Input: part model. Units: mm. Frame: model coordinates. A direction names the side the tool comes from. Round coordinates to 2 decimals unless told otherwise and drop trailing zeros. Loops run counter-clockwise (first coordinate to the right, second up) from the corner with the lowest first, then second, coordinate; pieces in that order, holes last. Notation, with made-up numbers: M 62.5,-23 L 120.5,-23 A13 ccw 120.5,-9 Z; hole C 37,40.5 d11. An arc over 180 degrees is marked long. Put each result on its own line as item: value. Start each with the question number.
1) Pin query (flat end, axial travel): pin 1 (5 mm diameter, centred on y = -0.5, z = -8, fed in from +X); pin 2 (2 mm diameter, centred on y = -3.5, z = -5.5, fed in from -X); pin 3 (5 mm diameter, centred on y = 4, z = -6, fed in from -X). Return the tip coordinate at first contact, or that it passes through.
2) Section C-C on x = -61.5. Output: boundary loops of the cut face in (y, z), plus the area to 3 significant figures.
3) Section A-A on y = 35. Output: boundary loops of the cut face in (x, z).
4) Reachability of faces 4 (the face through (-9.565, -40, -6)), 5 (the face through (-81, -3, -5)) from +Z, -Z, +X, -X, +Y, -Y: full face, straight path, thin tool, end or side. Return the list, or none.
5) Draft query along Y for faces 1 (the face through (-79, 20.744, -8)), 2 (the face through (-81, -38.396, -2)), 3 (the face through (-149.565, -40, -6)). Return one class per face: +Y half, -Y half, draft (parallel to the pull), parting line (faces both ways), or undercut.
6) Section D-D on z = -2.5. Output: boundary loops of the cut face in (x, y).
7) Section B-B on x = -84. Output: boundary loops of the cut face in (y, z).
8) Line query: probe 1 along Z at (x, y) = (-82, 14); probe 2 along Y at (x, z) = (-95.5, -3.5); probe 3 along Y at (x, z) = (-33, -7.5). Output: solid intervals per line, ascending.
from build123d import *

# Parameters (mm, degrees)
BOSS_EXTRUDE1_START = -10
BOSS_EXTRUDE1_DEPTH = 5
SKETCH1_3_W         = 140
SKETCH1_3_H         = 21.000815728
BOSS_EXTRUDE2_DEPTH = 10


with BuildPart() as part:
    # Sketch1 → Boss-Extrude1 (new body)
    with BuildSketch(Plane.XY.offset(BOSS_EXTRUDE1_START)):
        Polygon((-149.564743262, -9.396609427), (-149.564743262, -38.395793699), (-9.564743262, -38.395793699), (-9.564743262, -9.396609427), (-59.564743262, 50.603390573), (-99.564743262, 50.603390573), align=None)
        with BuildLine():
            Line((-72.064743262, 20.743540142), (-87.064743262, 20.743540142))
            ThreePointArc((-87.064743262, 20.743540142), (-79.564743262, 37.357918419), (-72.064743262, 20.743540142))
        make_face(mode=Mode.SUBTRACT)
    extrude(amount=BOSS_EXTRUDE1_DEPTH)

    # Sketch1<3> → Boss-Extrude2 (add)
    with BuildSketch(Plane.XY):
        with Locations((-79.564743262, -48.896201563)):
            Rectangle(SKETCH1_3_W, SKETCH1_3_H)
    extrude(amount=-BOSS_EXTRUDE2_DEPTH)


solid = part.part
Geometry results:
1. pin 1: stops at x = -14.9
1. pin 2: stops at x = -145.48
1. pin 3: stops at x = -140.48
2. outline: M -59.4,-10 L 50.6,-10 L 50.6,-5 L -38.4,-5 L -38.4,0 L -59.4,0 Z
2. area: 655 mm²
3. outline: M -112.57,-10 L -86.01,-10 L -86.01,-5 L -112.57,-5 Z; M -73.12,-10 L -46.56,-10 L -46.56,-5 L -73.12,-5 Z
4. face 4: +Z, -Z, +X, +Y, -Y
4. face 5: +Z, +X, -X, +Y
5. face 1: undercut
5. face 2: +Y half
5. face 3: draft
6. outline: M -149.56,-59.4 L -9.56,-59.4 L -9.56,-38.4 L -149.56,-38.4 Z
7. outline: M -59.4,-10 L 20.74,-10 L 20.74,-5 L -38.4,-5 L -38.4,0 L -59.4,0 Z; M 36.32,-10 L 50.6,-10 L 50.6,-5 L 36.32,-5 Z
8. probe 1: z = -10 to -5
8. probe 2: y = -59.4 to -38.4
8. probe 3: y = -59.4 to 18.73
